```python
from build123d import *

# Parameters (mm, degrees)
MODEL_R             = 1.25
BOSS_EXTRUDE1_DEPTH = 5


with BuildPart() as part:
    # Model → Boss-Extrude1 (new body)
    with BuildSketch(Plane.XY):
        Polygon((105.055071144, 3.719759624), (125.055071144, 23.719759624), (125.055071144, 53.719759624), (135.055071144, 63.719759624), (135.055071144, 103.719759624), (125.055071144, 113.719759624), (125.055071144, 143.719759624), (104.909839245, 163.864991523), (35.058830231, 163.723518711), (15.055071144, 143.719759624), (15.055071144, 113.719759624), (5.055071144, 103.719759624), (5.055071144, 63.719759624), (15.055071144, 53.719759624), (15.055071144, 23.719759624), (35.055071144, 3.719759624), align=None)
        with Locations((97.555071144, 6.219759624)):
            Circle(MODEL_R, mode=Mode.SUBTRACT)
        with Locations((122.555071144, 31.219759624)):
            Circle(MODEL_R, mode=Mode.SUBTRACT)
        with Locations((113.287304191, 15.487526577)):
            Circle(MODEL_R, mode=Mode.SUBTRACT)
        with Locations((42.555071144, 6.219759624)):
            Circle(MODEL_R, mode=Mode.SUBTRACT)
        with Locations((17.555071144, 31.219759624)):
            Circle(MODEL_R, mode=Mode.SUBTRACT)
        with Locations((26.822838097, 15.487526577)):
            Circle(MODEL_R, mode=Mode.SUBTRACT)
        with Locations((97.555071144, 161.219759624)):
            Circle(MODEL_R, mode=Mode.SUBTRACT)
        with Locations((122.555071144, 136.219759624)):
            Circle(MODEL_R, mode=Mode.SUBTRACT)
        with Locations((113.287304191, 151.951992671)):
            Circle(MODEL_R, mode=Mode.SUBTRACT)
        with Locations((42.555071144, 161.219759624)):
            Circle(MODEL_R, mode=Mode.SUBTRACT)
        with Locations((17.555071144, 136.219759624)):
            Circle(MODEL_R, mode=Mode.SUBTRACT)
        with Locations((26.822838097, 151.951992671)):
            Circle(MODEL_R, mode=Mode.SUBTRACT)
        with Locations((11.822838097, 60.487526577)):
            Circle(MODEL_R, mode=Mode.SUBTRACT)
        with Locations((7.555071144, 83.719759624)):
            Circle(MODEL_R, mode=Mode.SUBTRACT)
        with Locations((11.822838097, 106.951992671)):
            Circle(MODEL_R, mode=Mode.SUBTRACT)
        with Locations((128.287304191, 60.487526577)):
            Circle(MODEL_R, mode=Mode.SUBTRACT)
        with Locations((132.555071144, 83.719759624)):
            Circle(MODEL_R, mode=Mode.SUBTRACT)
        with Locations((128.287304191, 106.951992671)):
            Circle(MODEL_R, mode=Mode.SUBTRACT)
    extrude(amount=BOSS_EXTRUDE1_DEPTH)


solid = part.part
```
Geometry check sheet. Reference: the model listing, model coordinates, mm. A direction names the side the tool comes from. Coordinates: 2 decimals unless noted, no trailing zeros. Order: outer loops, then holes, each group sorted by start corner. A loop starts at its lowest first (then second) coordinate and runs counter-clockwise, first axis right, second up.
Q1. Thickness scan on probe 1 along Y at (x, z) = (97, 1.95); probe 2 along Y at (x, z) = (42, 1.25); probe 3 along X at (y, z) = (32.5, 0.75). Record the ranges inside material, lowest first.
Reply:
probe 1: y = 3.72 to 5.1, 7.34 to 160.1, 162.34 to 163.85
probe 2: y = 3.72 to 5.1, 7.34 to 160.1, 162.34 to 163.74
probe 3: x = 15.06 to 125.06
Q2. Sectioned sample at A-A on z = 1.2. Give the number of separate pieces and of enclosed holes in the cut face, and give its area (3 significant figures).
Reply:
separate pieces: 1
enclosed holes: 18
area: 17,700 mm2
Q3. Depth check by flat-ended pin: pin 1 Ø2.5 at (y, z) = (135.5, 2.5) entering from +X. Enter the tip coordinate at first touch or a pass-through.
Reply:
pin 1: stops at x = 125.06
Q4. Sectioned sample at C-C on x = 32. Record the cut outline in (y, z), and give its area (3 significant figures).
Reply:
outline: (6.77, 0) - (160.66, 0) - (160.66, 5) - (6.77, 5) - close
area: 769 mm2
Q5. Tool access check on faces 1 (the face through (15.055, 39, 2)), 2 (the face through (15.055, 129, 2)), 3 (the face through (125.055, 39, 2)), 4 (the face through (125.055, 129, 2)), 5 (the face through (5.055, 84, 2)). Record the directions out of +Z, -Z, +X, -X, +Y, -Y that give a thin tool (end or side, any length) a straight path to the whole face; none if there is none.
Reply:
face 1: +Z, -Z, -X, -Y
face 2: +Z, -Z, -X, +Y
face 3: +Z, -Z, +X, -Y
face 4: +Z, -Z, +X, +Y
face 5: +Z, -Z, -X, +Y, -Y
Q6. Sectioned sample at B-B on y = 50. Record the cut outline in (x, z).
Reply:
outline: (15.06, 0) - (125.06, 0) - (125.06, 5) - (15.06, 5) - close
